For this review, take the finished solid that the model builds, in its own axes (mm). A direction names the side the tool comes from. Round coordinates to 2 decimals unless told otherwise and drop trailing zeros. Order: outer loops, then holes, each group sorted by start corner. A loop starts at its lowest first (then second) coordinate and runs counter-clockwise, first axis right, second up. Notation, with made-up numbers: (32, 4) -> (70, 4) arc R25 ccw to (70, 17) -> close; hole circle Ø3 at (31.5, -13). An arc over 180 degrees is marked (long way). Use a Markdown table: item, result. Add a question column.
1) Machinability: for faces 4 (the face through (30, 15, 5)), 5 (the face through (14, 15, 14)), 6 (the face through (-7, -40.9, 40)), 7 (the face through (5, -24, 21.75)), which of the approach directions +Z, -Z, +X, -X, +Y, -Y give a long, thin tool a straight path to every point of the face, cutting with its end or side? Answer none if there is none.
2) Draft analysis for pull direction Z (two halves, no side actions). For faces 1 (the face through (3.99, -17.08, 61.22)), 2 (the face through (17.4, -10.9, 174.86)), 3 (the face through (5, -24, 15.75)), state which applies: pulls with the +Z half, pulls with the -Z half, needs draft (parallel to the pull), parting line crosses it, or undercut.
3) Clearance check with flat-ended pins moving along their axes: P1, Ø8, axis at y = 16, z = 72.5, coming from the +X side; P2, Ø5, axis at y = 3, z = 150, coming from the +X side; P3, Ø0.7, axis at x = 15.5, z = 62.5, coming from the +Y side; P4, Ø6, axis at x = 15.5, z = 184, coming from the +Y side (3 decimals). State where each tip first meets the part, or that it passes through.
4) Consider section B-B (z = 85). State the section outline as (x, y) points.
5) Consider section C-C (y = 3.5). State the section outline as (x, z) points.
6) Consider section A-A (x = 28). State the section outline as (y, z) points, plus the area to 3 significant figures.
7) Wall thickness on line 1 along Z through (x, y) = (-6.5, -35) (3 decimals); line 2 along Y through (x, z) = (15.53, 20.6); line 3 along Y through (x, z) = (21, 172): over which ranges is each line inside the solid? List them lowest first. Write a range as [from, to].
```python
from build123d import *

# Parameters (mm, degrees)
BOSS_EXTRUDE1_DEPTH     = 240
BOSS_EXTRUDE3_DEPTH     = 10
SKETCH5_R               = 1.75
CUT_EXTRUDE1_DEPTH      = 245.131112315
SKETCH6_W               = 7
SKETCH6_H               = 12
CUT_EXTRUDE2_DEPTH      = 21
SKETCH7_W               = 5
SKETCH7_H               = 240
BOSS_EXTRUDE4_DEPTH     = 54
SKETCH8_W               = 6
SKETCH8_H               = 6
BOSS_EXTRUDE5_DEPTH     = 24.4
CUT_EXTRUDE3_DEPTH      = 229.361692278
CUT_EXTRUDE3_DEPTH_BACK = 229.361692278
SKETCH9_R               = 1.7
SKETCH10_W              = 1.4
SKETCH10_H              = 6
CUT_EXTRUDE4_DEPTH      = 7
BOSS_EXTRUDE6_REACH     = 190.225
BOSS_EXTRUDE7_DEPTH     = 6
SKETCH13_R              = 3
BOSS_EXTRUDE8_DEPTH     = 30
SKETCH15_R              = 1.45
CUT_EXTRUDE5_DEPTH      = 5
SKETCH16_W              = 33.5
SKETCH16_H              = 33.5
CUT_EXTRUDE6_DEPTH      = 5
CHAMFER1_SIZE           = 10
CHAMFER1_SIZE_2         = 15


with BuildPart() as part:
    # Sketch1 → Boss-Extrude1 (new body)
    with BuildSketch(Plane.XY):
        Polygon((-10, 0), (0, 0), (0, 10), (10, 10), (10, 20), (-10, 20), align=None)
    extrude(amount=BOSS_EXTRUDE1_DEPTH)

    # Sketch4 → Boss-Extrude3 (add)
    with BuildSketch(Plane(origin=(0, 20, 0), x_dir=(1, 0, 0), z_dir=(0, 1, 0))):
        Polygon((10, 0), (40, 0), (40, -10), (18, -10), (10, -18), align=None)
    boss_extrude3 = extrude(amount=-BOSS_EXTRUDE3_DEPTH)

    # Sketch5 → Cut-Extrude1 (cut, through all)
    with BuildSketch(Plane(origin=(0, 0, 0), x_dir=(-1, 0, 0), z_dir=(0, 0, -1))):
        with Locations((-33, 15)):
            Circle(SKETCH5_R)
        with Locations((-23, 15)):
            Circle(SKETCH5_R)
    cut_extrude1 = extrude(amount=-CUT_EXTRUDE1_DEPTH, mode=Mode.SUBTRACT)

    # Sketch6 → Cut-Extrude2 (cut)
    with BuildSketch(Plane(origin=(40, 0, 0), x_dir=(0, 0, -1), z_dir=(1, 0, 0))):
        with Locations((-8.5, 15)):
            Rectangle(SKETCH6_W, SKETCH6_H)
    cut_extrude2 = extrude(amount=-CUT_EXTRUDE2_DEPTH, mode=Mode.SUBTRACT)

    # Mirror1: Boss-Extrude3, Cut-Extrude1, Cut-Extrude2 across plane
    add(boss_extrude3.mirror(Plane(origin=(0, 0, 120), x_dir=(1, 0, 0), z_dir=(0, 0, -1))))
    add(cut_extrude1.mirror(Plane(origin=(0, 0, 120), x_dir=(1, 0, 0), z_dir=(0, 0, -1))), mode=Mode.SUBTRACT)
    add(cut_extrude2.mirror(Plane(origin=(0, 0, 120), x_dir=(1, 0, 0), z_dir=(0, 0, -1))), mode=Mode.SUBTRACT)

    # Sketch7 → Boss-Extrude4 (add)
    with BuildSketch(Plane.XZ):
        with Locations((-7.5, 120)):
            Rectangle(SKETCH7_W, SKETCH7_H)
    extrude(amount=BOSS_EXTRUDE4_DEPTH)

    # Sketch8 → Boss-Extrude5 (add)
    with BuildSketch(Plane(origin=(-5, 0, 0), x_dir=(0, 0, -1), z_dir=(1, 0, 0))):
        with Locations((-18.75, -24.15)):
            Rectangle(SKETCH8_W, SKETCH8_H)
        with Locations((-61.18, -24.15)):
            Rectangle(SKETCH8_W, SKETCH8_H)
    extrude(amount=BOSS_EXTRUDE5_DEPTH)

    # Sketch9 → Cut-Extrude3 (cut, two sides: drawn at the far end of the back side and taken through both)
    with BuildSketch(Plane.XY.offset(21.75).offset(-CUT_EXTRUDE3_DEPTH_BACK)):
        with Locations((15.53, -24.25)):
            Circle(SKETCH9_R)
    extrude(amount=CUT_EXTRUDE3_DEPTH + CUT_EXTRUDE3_DEPTH_BACK, mode=Mode.SUBTRACT)

    # Sketch10 → Cut-Extrude4 (cut)
    with BuildSketch(Plane(origin=(19.4, 0, 0), x_dir=(0, 0, -1), z_dir=(1, 0, 0))):
        with Locations((-18.75, -24.15)):
            Rectangle(SKETCH10_W, SKETCH10_H)
        with Locations((-61.18, -24.15)):
            Rectangle(SKETCH10_W, SKETCH10_H)
    extrude(amount=-CUT_EXTRUDE4_DEPTH, mode=Mode.SUBTRACT)

    # Boss-Extrude6: up to this face of the body (flat: up to its plane)
    boss_extrude6_end = Plane(part.part.faces().sort_by_distance((6.649247597, -24.143388326, 58.18))[0])
    # Sketch11 → Boss-Extrude6 (add, up to the picked face)
    with BuildSketch(Plane.XY.offset(64.18), mode=Mode.PRIVATE) as boss_extrude6_sk1:
        Polygon((12.722534603, -21.15), (-5, -12.885846393), (-5, -17.885846393), (2, -21.15), align=None)
    boss_extrude6_tool1 = split(extrude(boss_extrude6_sk1.sketch, amount=-BOSS_EXTRUDE6_REACH, mode=Mode.PRIVATE), bisect_by=boss_extrude6_end, keep=Keep.BOTH, mode=Mode.PRIVATE)
    # Sketch11 → Boss-Extrude6 (add, up to the picked face)
    with BuildSketch(Plane.XY.offset(64.18), mode=Mode.PRIVATE) as boss_extrude6_sk2:
        Polygon((-5, -30.414153607), (2, -27.15), (12.722534603, -27.15), (-5, -35.414153607), align=None)
    boss_extrude6_tool2 = split(extrude(boss_extrude6_sk2.sketch, amount=-BOSS_EXTRUDE6_REACH, mode=Mode.PRIVATE), bisect_by=boss_extrude6_end, keep=Keep.BOTH, mode=Mode.PRIVATE)
    add(boss_extrude6_tool1.solids().sort_by(Axis((1.568177, -18.087209, 64.18), (0, 0, -1)))[0])
    add(boss_extrude6_tool2.solids().sort_by(Axis((1.568177, -30.212791, 64.18), (0, 0, -1)))[0])

    # Sketch12 → Boss-Extrude7 (add)
    with BuildSketch(Plane(origin=(0, 0, 15.75), x_dir=(-1, 0, 0), z_dir=(0, 0, -1))):
        Polygon((-12.722534603, -21.15), (-2, -21.15), (5, -17.885846393), (5, -12.885846393), align=None)
        Polygon((-2, -27.15), (-12.722534603, -27.15), (5, -35.414153607), (5, -30.414153607), align=None)
    extrude(amount=-BOSS_EXTRUDE7_DEPTH)

    # Sketch13 → Boss-Extrude8 (add)
    with BuildSketch(Plane(origin=(-5, 0, 0), x_dir=(0, 0, -1), z_dir=(1, 0, 0))):
        with Locations(Location((-230, -10, 0), (0, 0, 180))):
            Circle(SKETCH13_R)
        with Locations(Location((-172, -10, 0), (0, 0, 180))):
            Circle(SKETCH13_R)
    extrude(amount=BOSS_EXTRUDE8_DEPTH)

    # Sketch15 → Cut-Extrude5 (cut)
    with BuildSketch(Plane(origin=(25, 0, 0), x_dir=(0, 0, -1), z_dir=(1, 0, 0))):
        with Locations((-230, -10)):
            Circle(SKETCH15_R)
        with Locations((-172, -10)):
            Circle(SKETCH15_R)
    extrude(amount=-CUT_EXTRUDE5_DEPTH, mode=Mode.SUBTRACT)

    # Sketch16 → Cut-Extrude6 (cut)
    with BuildSketch(Plane(origin=(-5, 0, 0), x_dir=(0, 0, -1), z_dir=(1, 0, 0))):
        with Locations((-39.965, -24.15)):
            Rectangle(SKETCH16_W, SKETCH16_H)
    extrude(amount=-CUT_EXTRUDE6_DEPTH, mode=Mode.SUBTRACT)

    # Chamfer1
    # the kernel refuses this chamfer: 15, 10 mm, written as the material it adds along each edge
    with BuildSketch(Plane(origin=(-5, -10, 172), x_dir=(0, 0, 1), z_dir=(0, 1, 0))) as chamfer1_piece_1:
        Polygon((3 + CHAMFER1_SIZE, 0), (3, CHAMFER1_SIZE_2), (3, 0), align=None)
    revolve(axis=Axis((-5, -10, 172), (1, 0, 0)))
    with BuildSketch(Plane(origin=(-5, -10, 230), x_dir=(0, 0, 1), z_dir=(0, 1, 0))) as chamfer1_piece_2_section:
        Polygon((3 + CHAMFER1_SIZE, 0), (3, CHAMFER1_SIZE_2), (3, 0), align=None)
    chamfer1_piece_2 = revolve(axis=Axis((-5, -10, 230), (1, 0, 0)), mode=Mode.PRIVATE)
    chamfer1_piece_2 = split(chamfer1_piece_2, bisect_by=Plane(origin=(2.41807783, -10, 240), z_dir=(0, 0, -1)), keep=Keep.TOP, mode=Mode.PRIVATE)
    add(chamfer1_piece_2)


solid = part.part
```
Results list:
| question | item | result |
|---|---|---|
| 1 | face 4 | +X, +Y, -Y |
| 1 | face 5 | +X, +Y |
| 1 | face 6 | +X, -X |
| 1 | face 7 | +X, -Y |
| 2 | face 1 | needs draft |
| 2 | face 2 | undercut |
| 2 | face 3 | pulls with the -Z half |
| 3 | P1 | x = 10 |
| 3 | P2 | x = 0 |
| 3 | P3 | y = -21.15 |
| 3 | P4 | through |
| 4 | outline | (-10, -54) -> (-5, -54) -> (-5, 0) -> (0, 0) -> (0, 10) -> (10, 10) -> (10, 20) -> (-10, 20) -> close |
| 5 | outline | (-10, 0) -> (0, 0) -> (0, 240) -> (-10, 240) -> close |
| 6 | outline | (10, 0) -> (20, 0) -> (20, 5) -> (10, 5) -> close; (10, 235) -> (20, 235) -> (20, 240) -> (10, 240) -> close |
| 6 | area | 100 mm2 |
| 7 | line 1 | [0, 23.215], [56.715, 240] |
| 7 | line 2 | [-27.15, -25.95], [-22.55, -21.15] |
| 7 | line 3 | [-13, -11.45], [-8.55, -7] |
